CAD build for the part. Positions are in the model's coordinates, mm. A direction names the side the tool comes from. Give positions to 0.01 mm unless a question says otherwise; leave off trailing zeros. Order: outer loops, then holes, each group sorted by start corner. A loop starts at its lowest first (then second) coordinate and runs counter-clockwise, first axis right, second up. Notation, with made-up numbers: M -36.75,31.5 L -1.75,31.5 A17 ccw -1.75,55.5 Z; hole C 12.25,-39 d6. An arc over 180 degrees is marked long. Put each result on its own line as item: value. Start each with the question number.
1) Drill centre lines: line 1 (X direction, y = -0.6, z = 0); line 2 (X direction, y = -2.5, z = 0); line 3 (Y direction, x = -0.5, z = 5.5). Where is each one in solid material? Low to high. Write a range as [from, to].
2) Cut at B-B (z = 0). Write the cut outline in (x, y), and give its area (3 significant figures).
3) Cut at D-D (y = -2.95). Write the cut outline in (x, z).
4) Tool access for faces 4 (the face through (1.352, -2.986, -4.292)), 5 (the face through (-2, -4, 0)), 6 (the face through (-1.952, 0.493, -0.434)): list every direction of +Z, -Z, +X, -X, +Y, -Y with a clear straight run to the whole face (end or side of a thin tool).
5) Cut at C-C (y = -0.6). Write the cut outline in (x, z), and give its area (3 significant figures).
6) Two-plate mould, pull along X, no slides. Class faces 1 (the face through (-0.45, -1.54, -1.43)), 2 (the face through (3.604, -0.986, 11.446)), 3 (the face through (0, -2, 5)): released by +X, released by -X, zero draft, split by the parting line, or undercut.
7) Pin check, flat tips, straight feed: pin 1 (4 mm diameter, centred on x = -4, z = -6.5, fed in from -Y); pin 2 (1.5 mm diameter, centred on x = 4, y = -3, fed in from -Z). Stop position of each tip, or through.
8) Cut at A-A (x = 0). Write the cut outline in (y, z).
```python
from build123d import *

# Parameters (mm, degrees)
SKETCH1_R           = 12
BOSS_EXTRUDE1_DEPTH = 2
SKETCH2_R           = 4.5
BOSS_EXTRUDE2_DEPTH = 2
SKETCH3_R           = 1.5
CUT_EXTRUDE1_DEPTH  = 18.435595774
SKETCH4_R           = 2
SKETCH4_R_2         = 1.5
BOSS_EXTRUDE3_DEPTH = 1


with BuildPart() as part:
    # Sketch1 → Boss-Extrude1 (new body)
    with BuildSketch(Plane(origin=(0, 0, 0), x_dir=(1, 0, 0), z_dir=(0, 1, 0))):
        with Locations(Location((0, 0, 0), (0, 0, 270))):
            Circle(SKETCH1_R)
    extrude(amount=-BOSS_EXTRUDE1_DEPTH)

    # Sketch2 → Boss-Extrude2 (add)
    with BuildSketch(Plane.XZ.offset(2)):
        with Locations(Location((0, 0, 0), (0, 0, 270))):
            Circle(SKETCH2_R)
    extrude(amount=BOSS_EXTRUDE2_DEPTH)

    # Sketch3 → Cut-Extrude1 (cut, through all)
    with BuildSketch(Plane.XZ.offset(4)):
        with Locations(Location((0, 0, 0), (0, 0, 270))):
            Circle(SKETCH3_R)
    extrude(amount=-CUT_EXTRUDE1_DEPTH, mode=Mode.SUBTRACT)

    # Sketch4 → Boss-Extrude3 (add)
    with BuildSketch(Plane(origin=(0, 0, 0), x_dir=(1, 0, 0), z_dir=(0, 1, 0))):
        with Locations(Location((0, 0, 0), (0, 0, 270))):
            Circle(SKETCH4_R)
        with Locations(Location((0, 0, 0), (0, 0, 90))):
            Circle(SKETCH4_R_2, mode=Mode.SUBTRACT)
    extrude(amount=BOSS_EXTRUDE3_DEPTH)


solid = part.part
```
Solution:
1. line 1: [-12, -1.5], [1.5, 12]
1. line 2: [-4.5, -1.5], [1.5, 4.5]
1. line 3: [-2, 0]
2. outline: M -12,-2 L -4.5,-2 L -4.5,-4 L -1.5,-4 L -1.5,1 L -2,1 L -2,0 L -12,0 Z; M 1.5,-4 L 4.5,-4 L 4.5,-2 L 12,-2 L 12,0 L 2,0 L 2,1 L 1.5,1 Z
2. area: 55.0 mm²
3. outline: C 0,0 d9; hole C 0,0 d3
4. face 4: -Y
4. face 5: +Z, -Z, +X, -X, -Y
4. face 6: +Y
5. outline: C 0,0 d24; hole C 0,0 d3
5. area: 445 mm²
6. face 1: undercut
6. face 2: split by the parting line
6. face 3: zero draft
7. pin 1: y = -2
7. pin 2: z = -3.11
8. outline: M -4,-4.5 L -2,-4.5 L -2,-12 L 0,-12 L 0,-2 L 1,-2 L 1,-1.5 L -4,-1.5 Z; M -4,1.5 L 1,1.5 L 1,2 L 0,2 L 0,12 L -2,12 L -2,4.5 L -4,4.5 Z
